Could you check a few things on this model? Use its own coordinates, in mm. A direction names the side the tool comes from. Round coordinates to 2 decimals unless told otherwise and drop trailing zeros. Loops run counter-clockwise (first coordinate to the right, second up) from the corner with the lowest first, then second, coordinate; pieces in that order, holes last.
from build123d import *

# Parameters (mm, degrees)
BASPROSKE_W                  = 10
BASPROSKE_H                  = 6
TOOTHCUT_DEPTH               = 14.114877049
TEETHCUTS_COUNT              = 10
TEETHCUTS_ANGLE              = 324
BORSKE_R                     = 0.4
BORE_DEPTH                   = 50.0000508
CROQUIS1_R                   = 3.75
SALIENTE_EXTRUIR1_DEPTH      = 10
TALADRO_DE_MARGEN_PARA_M51_D = 5.3
SALIENTE_EXTRUIR2_DEPTH      = 10


with BuildPart() as part:
    # BasProSke → Base-Revolve (revolve)
    with BuildSketch(Plane(origin=(0, 0, 0), x_dir=(1, 0, 0), z_dir=(0, 1, 0)), mode=Mode.PRIVATE) as base_revolve_sk:
        with Locations((5, 3)):
            Rectangle(BASPROSKE_W, BASPROSKE_H)
    revolve(base_revolve_sk.sketch.rotate(Axis((-10, 0, 0), (1, 0, 0)), 180), axis=Axis((-10, 0, 0), (1, 0, 0)))

    # TooCutSke → ToothCut (cut, through all)
    with BuildSketch(Plane(origin=(0, 0, 0), x_dir=(0, 0, -1), z_dir=(1, 0, 0))):
        with BuildLine():
            ThreePointArc((0.59278292, 3.701838653), (0, 3.749), (-0.59278292, 3.701838653))
            ThreePointArc((-0.59278292, 3.701838653), (-0.846593509, 4.924114224), (-1.775771316, 5.757784417))
            ThreePointArc((-1.775771316, 5.757784417), (0, 6.0254), (1.775771316, 5.757784417))
            ThreePointArc((1.775771316, 5.757784417), (0.846593509, 4.924114224), (0.59278292, 3.701838653))
        make_face()
    toothcut = extrude(amount=TOOTHCUT_DEPTH, mode=Mode.SUBTRACT)

    # TeethCuts: ToothCut ×10 about axis
    teethcuts_axis = Axis((-10, 0, 0), (1, 0, 0))
    for i in range(1, TEETHCUTS_COUNT):
        add(toothcut.rotate(teethcuts_axis, i * TEETHCUTS_ANGLE / (TEETHCUTS_COUNT - 1)), mode=Mode.SUBTRACT)

    # BorSke → Bore (cut, symmetric)
    with BuildSketch(Plane(origin=(0, 0, 0), x_dir=(0, 0, -1), z_dir=(1, 0, 0))):
        with Locations(Location((0, 0, 0), (0, 0, 180))):
            Circle(BORSKE_R)
    extrude(amount=BORE_DEPTH, both=True, mode=Mode.SUBTRACT)

    # Croquis1 → Saliente-Extruir1 (add)
    with BuildSketch(Plane.ZY):
        with Locations(Location((0, 0, 0), (0, 0, 188.906595326))):
            Circle(CROQUIS1_R)
    extrude(amount=SALIENTE_EXTRUIR1_DEPTH)

    # Taladro de margen para M51 (through all)
    with Locations(Plane.ZY.offset(10)):
        with Locations((0, 0)):
            Hole(TALADRO_DE_MARGEN_PARA_M51_D / 2)

    # Croquis5 → Saliente-Extruir2 (add)
    with BuildSketch(Plane(origin=(10, 0, 0), x_dir=(0, 0, -1), z_dir=(1, 0, 0))):
        with BuildLine():
            Line((2.149418526, 0), (2.149418526, 1.55))
            ThreePointArc((2.149418526, 1.55), (2.65, 0), (2.149418526, -1.55))
            Line((2.149418526, -1.55), (2.149418526, 0))
        make_face()
    extrude(amount=-SALIENTE_EXTRUIR2_DEPTH)


solid = part.part
Item 1: Will these pins go through, and if not, where does the flat tip stop? pin 1 (3 mm diameter, centred on x = -7, y = -2, fed in from +Z); pin 2 (1 mm diameter, centred on x = 2.5, y = -1.5, fed in from -Z); pin 3 (0.8 mm diameter, centred on y = 5, z = -1, fed in from -X); pin 4 (4 mm diameter, centred on y = 3, z = 2.5, fed in from -X).
Results list:
pin 1: stops at z = 3.72
pin 2: stops at z = -4.04
pin 3: stops at x = 0
pin 4: stops at x = -10
Item 2: If we section it at D-D, the plane x = -4.5: Please give me the cut outline in (y, z), then the cut area to 3 significant figures.
Results list:
outline: circle Ø7.5 at (0, 0); hole circle Ø5.3 at (0, 0)
area: 22.1 mm2
Item 3: For faces 4 (the flat face through (0, 4.5, 1.4)), 5 (the flat face through (0, 4.5, -1.4)), 6 (the flat face through (0, -3, 4)), which set-ups out of +Z, -Z, +X, -X, +Y, -Y let a thin tool reach every point of the face, with its end or its side?
Results list:
face 4: +Z, -X, +Y
face 5: -Z, -X, +Y
face 6: +Z, -X, -Y
Item 4: We'd pull the mould along Z, two halves only. Please class faces 1 (the cylindrical face through (-4.93, 3.743, 0.236)), 2 (the flat face through (-10, -3, 0)), 3 (the cylindrical face through (4.93, -3.471, -3.546)): released by +Z, released by -Z, zero draft, split by the parting line, or undercut.
Results list:
face 1: split by the parting line
face 2: zero draft
face 3: undercut
Item 5: If we section it at B-B, the plane y = -5: Please give me the cut outline in (x, z).
Results list:
outline: (0, -2.2) - (10, -2.2) - (10, -0.89) - (0, -0.89) - close; (0, 0.89) - (10, 0.89) - (10, 2.2) - (0, 2.2) - close
Item 6: If I drill on line 1 along Y through (x, z) = (2.75, 4.25); line 2 along Z through (x, y) = (7, -2.75); line 3 along Z through (x, y) = (3.5, 0), over which ranges is the centre line in solid material (lowest first)?
Results list:
line 1: y = -3.65 to -2.16, -0.74 to 0.74, 2.16 to 3.65
line 2: z = -4.71 to -2.72, -2.55 to 2.55, 2.72 to 4.71
line 3: z = -6 to -2.15, 2.65 to 6
Item 7: If we section it at C-C, the plane z = 4.25: Please give me the cut outline in (x, y).
Results list:
outline: (0, -3.65) - (10, -3.65) - (10, -2.16) - (0, -2.16) - close; (0, -0.74) - (10, -0.74) - (10, 0.74) - (0, 0.74) - close; (0, 2.16) - (10, 2.16) - (10, 3.65) - (0, 3.65) - close
